Here's how the part is built. I have some questions about the finished solid (model axes, mm). A direction names the side the tool comes from. Coordinates: 2 decimals unless noted, no trailing zeros. Write each loop counter-clockwise with the first axis right and the second up, starting at its lowest first coordinate (ties: lowest second). Pieces come first, ordered by that corner, then holes.
Item 1: If I drill on line 1 (Z direction, x = 50, y = 4.95); line 2 (Z direction, x = -38.1, y = 3.4) (3 decimals); line 3 (X direction, y = 3.15, z = -25.5), over which ranges is the centre line in solid material (lowest first)?
Item 2: We'd pull the mould along X, two halves only. Please class faces 1 (the face through (-1, 3, 35)), 2 (the face through (60, 3, 0)), 3 (the face through (-38.654, 3.042, -22.906)): +X half, -X half, draft (parallel to the pull), parting line (faces both ways), or undercut.
Item 3: If we section it at A-A (x = 50): Please give me the cut outline in (y, z), then the cut area to 3 significant figures.
Item 4: For faces 4 (the face through (51.34, 4.99, -27.11)), 5 (the face through (54.032, 1.972, -31.324)), which set-ups out of +Z, -Z, +X, -X, +Y, -Y let a thin tool reach every point of the face, with its end or its side?
Item 5: I'm going to push flat-ended pins straight in: pin 1 Ø4.5 at (x, z) = (51, -22.5) entering from -Y; pin 2 Ø3 at (x, z) = (-50, -25) entering from -Y. Where does each tip first touch, or does it pass through?
Item 6: If we section it at B-B (y = 1.75): Count the separate pieces of the cut face and the enclosed holes in it, then the cut area to 3 significant figures.
from build123d import *

# Parameters (mm, degrees)
SKETCH1_W           = 120
SKETCH1_H           = 70
SKETCH1_R           = 2.5
BOSS_EXTRUDE1_DEPTH = 6
SKETCH2_R           = 2.555
CUT_EXTRUDE1_DEPTH  = 7
SKETCH3_R           = 7.5
CUT_EXTRUDE2_DEPTH  = 4


with BuildPart() as part:
    # Sketch1 → Boss-Extrude1 (new body)
    with BuildSketch(Plane(origin=(0, 0, 0), x_dir=(1, 0, 0), z_dir=(0, 1, 0))):
        Rectangle(SKETCH1_W, SKETCH1_H)
        with Locations((-50, -25)):
            Circle(SKETCH1_R, mode=Mode.SUBTRACT)
        with Locations((-50, 25)):
            Circle(SKETCH1_R, mode=Mode.SUBTRACT)
        with Locations((50, 25)):
            Circle(SKETCH1_R, mode=Mode.SUBTRACT)
        with Locations((50, -25)):
            Circle(SKETCH1_R, mode=Mode.SUBTRACT)
    extrude(amount=BOSS_EXTRUDE1_DEPTH)

    # Sketch2 → Cut-Extrude1 (cut, through all)
    with BuildSketch(Plane(origin=(0, 6, 0), x_dir=(1, 0, 0), z_dir=(0, 1, 0))):
        with Locations((38.1, -25.4)):
            Circle(SKETCH2_R)
        with Locations((-38.1, -25.4)):
            Circle(SKETCH2_R)
        with Locations((38.1, 25.4)):
            Circle(SKETCH2_R)
        with Locations((-38.1, 25.4)):
            Circle(SKETCH2_R)
    extrude(amount=-CUT_EXTRUDE1_DEPTH, mode=Mode.SUBTRACT)

    # Sketch3 → Cut-Extrude2 (cut)
    with BuildSketch(Plane(origin=(0, 0, 0), x_dir=(1, 0, 0), z_dir=(0, 1, 0))):
        with Locations((-50, 25)):
            Circle(SKETCH3_R)
        with Locations((50, 25)):
            Circle(SKETCH3_R)
        with Locations((50, -25)):
            Circle(SKETCH3_R)
        with Locations((-50, -25)):
            Circle(SKETCH3_R)
    extrude(amount=CUT_EXTRUDE2_DEPTH, mode=Mode.SUBTRACT)


solid = part.part
Answer list:
1. line 1: z = -35 to -27.5, -22.5 to 22.5, 27.5 to 35
1. line 2: z = -35 to -27.955, -22.845 to 22.845, 27.955 to 35
1. line 3: x = -60 to -57.48, -42.52 to -40.65, -35.55 to 35.55, 40.65 to 42.52, 57.48 to 60
2. face 1: draft
2. face 2: +X half
2. face 3: undercut
3. outline: (0, -35) - (6, -35) - (6, -27.5) - (4, -27.5) - (4, -32.5) - (0, -32.5) - close; (0, -17.5) - (4, -17.5) - (4, -22.5) - (6, -22.5) - (6, 22.5) - (4, 22.5) - (4, 17.5) - (0, 17.5) - close; (0, 32.5) - (4, 32.5) - (4, 27.5) - (6, 27.5) - (6, 35) - (0, 35) - close
3. area: 280 mm2
4. face 4: +Y, -Y
4. face 5: -Y
5. pin 1: stops at y = 4
5. pin 2: passes through
6. separate pieces: 1
6. enclosed holes: 8
6. area: 7,610 mm2
